Geometry check sheet. Reference: the model listing, model coordinates, mm. Face numbers are marked on the shaded views. Round coordinates to 2 decimals unless told otherwise and drop trailing zeros. Loops run counter-clockwise (first coordinate to the right, second up) from the corner with the lowest first, then second, coordinate; pieces in that order, holes last.
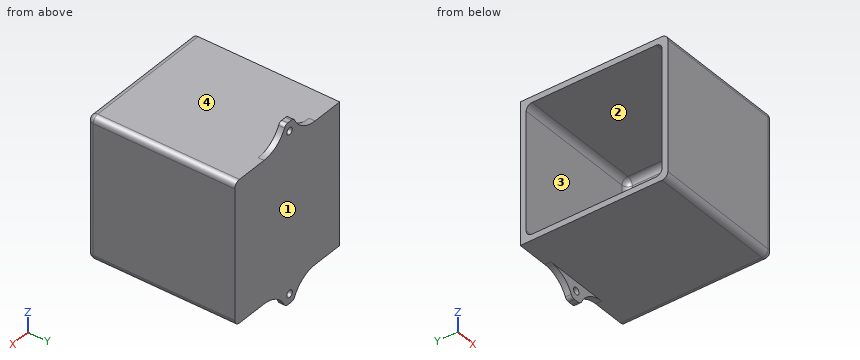
```python
from build123d import *

# Parameters (mm, degrees)
SKETCH1_W           = 60
SKETCH1_H           = 60
BOSS_EXTRUDE1_DEPTH = 60
SHELL1_T            = -2.5
SKETCH5_R           = 1.5
BOSS_EXTRUDE3_DEPTH = 2.5
SKETCH6_W           = 60
SKETCH6_H           = 60
BOSS_EXTRUDE4_DEPTH = 2.5
SKETCH7_W           = 60
SKETCH7_H           = 62.5
CUT_EXTRUDE1_DEPTH  = 2.5
FILLET4_R           = 2.5
FILLET5_R           = 12.5
FILLET6_R           = 2.5


with BuildPart() as part:
    # Sketch1 → Boss-Extrude1 (new body)
    with BuildSketch(Plane(origin=(0, 0, 0), x_dir=(1, 0, 0), z_dir=(0, 1, 0))):
        with Locations((30, 30)):
            Rectangle(SKETCH1_W, SKETCH1_H)
    extrude(amount=BOSS_EXTRUDE1_DEPTH)

    # Shell1
    shell1_openings = [part.faces().sort_by_distance(p)[0] for p in [
        (30, 0, -30),
    ]]
    offset(amount=SHELL1_T, openings=shell1_openings, kind=Kind.INTERSECTION)

    # Sketch5 → Boss-Extrude3 (add)
    # profile 1 of 2: a face of its own
    with BuildSketch(Plane(origin=(0, 60, 0), x_dir=(1, 0, 0), z_dir=(0, 1, 0))):
        with BuildLine():
            Line((27, 60), (27, 66))
            ThreePointArc((27, 66), (27.585786438, 67.414213562), (29, 68))
            Line((29, 68), (31, 68))
            ThreePointArc((31, 68), (32.414213562, 67.414213562), (33, 66))
            Line((33, 66), (33, 60))
            Line((33, 60), (27, 60))
        make_face()
        with Locations(Location((30, 64, 0), (0, 0, 270))):
            Circle(SKETCH5_R, mode=Mode.SUBTRACT)
    # profile 2 of 2: a face of its own
    with BuildSketch(Plane(origin=(0, 60, 0), x_dir=(1, 0, 0), z_dir=(0, 1, 0))):
        with BuildLine():
            Line((33, 0), (27, 0))
            Line((27, 0), (27, -6))
            ThreePointArc((27, -6), (27.585786438, -7.414213562), (29, -8))
            Line((29, -8), (31, -8))
            ThreePointArc((31, -8), (32.414213562, -7.414213562), (33, -6))
            Line((33, -6), (33, 0))
        make_face()
        with Locations(Location((30, -4, 0), (0, 0, 90))):
            Circle(SKETCH5_R, mode=Mode.SUBTRACT)
    extrude(amount=-BOSS_EXTRUDE3_DEPTH)

    # Sketch6 → Boss-Extrude4 (add)
    with BuildSketch(Plane.XZ):
        with Locations((30, -30)):
            Rectangle(SKETCH6_W, SKETCH6_H)
    extrude(amount=BOSS_EXTRUDE4_DEPTH)

    # Sketch7 → Cut-Extrude1 (cut)
    with BuildSketch(Plane.ZY):
        with Locations((-30, 28.75)):
            Rectangle(SKETCH7_W, SKETCH7_H)
    extrude(amount=-CUT_EXTRUDE1_DEPTH, mode=Mode.SUBTRACT)

    # Fillet4
    fillet4_edges = [part.edges().sort_by_distance(p)[0] for p in [
        (31.25, -2.5, 0),
        (60, -2.5, -30),
        (31.25, -2.5, -60),
        (60, 28.75, -60),
        (60, 28.75, 0),
    ]]
    fillet(fillet4_edges, radius=FILLET4_R)

    # Fillet5
    # the kernel refuses this fillet: 12.5 mm, written as the material it adds along each edge
    with BuildSketch(Plane(origin=(27, 60, 0), x_dir=(-1, 0, 0), z_dir=(0, -1, 0)), Plane(origin=(33, 60, -60), x_dir=(1, 0, 0), z_dir=(0, -1, 0))) as fillet5_piece_1:
        with BuildLine():
            CenterArc((10.961481397, -12.5), FILLET5_R, 90, 63.366881251)
            Line((-0.212209463, -6.896551724), (-1.329578548, -6.336206897))
            ThreePointArc((-1.329578548, -6.336206897), (-1.25, -6), (-1.25, 0))
            Line((-1.25, 0), (0, 1.25))
            Line((0, 1.25), (10.961481397, 1.25))
            Line((10.961481397, 1.25), (10.961481397, 0))
        make_face()
    extrude(amount=2.5)
    with BuildSketch(Plane(origin=(33, 60, 0), x_dir=(1, 0, 0), z_dir=(0, -1, 0)), Plane(origin=(27, 60, -60), x_dir=(-1, 0, 0), z_dir=(0, -1, 0))) as fillet5_piece_2:
        with BuildLine():
            CenterArc((10.961481397, 12.5), FILLET5_R, 206.633118749, 63.366881251)
            Line((-0.212209463, 6.896551724), (-1.329578548, 6.336206897))
            ThreePointArc((-1.329578548, 6.336206897), (-1.25, 6), (-1.25, 0))
            Line((-1.25, 0), (0, -1.25))
            Line((0, -1.25), (10.961481397, -1.25))
            Line((10.961481397, -1.25), (10.961481397, 0))
        make_face()
    extrude(amount=2.5)

    # Fillet6
    fillet6_edges = [part.edges().sort_by_distance(p)[0] for p in [
        (30, 0, -2.5),
        (57.5, 0, -30),
        (57.5, 28.75, -2.5),
        (30, 0, -57.5),
        (57.5, 28.75, -57.5),
        (30, 57.5, -2.5),
        (57.5, 57.5, -30),
        (30, 57.5, -57.5),
    ]]
    fillet(fillet6_edges, radius=FILLET6_R)


solid = part.part
```
1) Scan lines: line 1 along Y through (x, z) = (26, -21.5); line 2 along Z through (x, y) = (21, 5.5); line 3 along X through (y, z) = (3, -12). Record each from-to range of solid material in increasing order.
Report:
line 1: y = -2.5 to 0, 57.5 to 60
line 2: z = -60 to -57.5, -2.5 to 0
line 3: x = 57.5 to 60
2) Mould release check, pull along Z, two halves, no side actions. Record for the marked faces 1, 2, 3 and 4: +Z half, -Z half, draft (parallel to the pull), parting line (faces both ways), or undercut.
Report:
face 1: draft
face 2: undercut
face 3: undercut
face 4: +Z half
3) Sectioned sample at C-C, the plane x = 49. Record the cut outline in (y, z).
Report:
outline: (-2.5, -57.5) arc R2.5 ccw to (0, -60) - (60, -60) - (60, 0) - (0, 0) arc R2.5 ccw to (-2.5, -2.5) - close; hole (0, -55) arc R2.5 ccw to (2.5, -57.5) - (55, -57.5) arc R2.5 ccw to (57.5, -55) - (57.5, -5) arc R2.5 ccw to (55, -2.5) - (2.5, -2.5) arc R2.5 ccw to (0, -5) - close
4) Gauge pin test, flat ends, axial feed: pin 1 (5 mm diameter, centred on x = 30, z = 4, fed in from -Y); pin 2 (16.5 mm diameter, centred on x = 32.5, y = 37, fed in from +Z); pin 3 (25 mm diameter, centred on y = 40, z = -26, fed in from -X); pin 4 (1.8 mm diameter, centred on x = 30, z = -64, fed in from -Y). Record the tip position at first contact, or that the pin passes through.
Report:
pin 1: stops at y = 57.5
pin 2: stops at z = 0
pin 3: stops at x = 57.5
pin 4: passes through
5) Sectioned sample at D-D, the plane z = -32. Record the cut outline in (x, y).
Report:
outline: (2.5, -2.5) - (57.5, -2.5) arc R2.5 ccw to (60, 0) - (60, 60) - (2.5, 60) - (2.5, 57.5) - (55, 57.5) arc R2.5 cw to (57.5, 55) - (57.5, 2.5) arc R2.5 cw to (55, 0) - (2.5, 0) - close
6) Sectioned sample at B-B, the plane y = 43.5. Record the cut outline in (x, z).
Report:
outline: (2.5, -60) - (57.5, -60) arc R2.5 ccw to (60, -57.5) - (60, -2.5) arc R2.5 ccw to (57.5, 0) - (2.5, 0) - (2.5, -2.5) - (55, -2.5) arc R2.5 cw to (57.5, -5) - (57.5, -55) arc R2.5 cw to (55, -57.5) - (2.5, -57.5) - close
7) Sectioned sample at A-A, the plane x = 30. Record the cut outline in (y, z), then the cut area to 3 significant figures.
Report:
outline: (-2.5, -57.5) arc R2.5 ccw to (0, -60) - (57.5, -60) - (57.5, -62.5) - (60, -62.5) - (60, 2.5) - (57.5, 2.5) - (57.5, 0) - (0, 0) arc R2.5 ccw to (-2.5, -2.5) - close; (57.5, -68) - (60, -68) - (60, -65.5) - (57.5, -65.5) - close; (57.5, 5.5) - (60, 5.5) - (60, 8) - (57.5, 8) - close; hole (0, -55) arc R2.5 ccw to (2.5, -57.5) - (55, -57.5) arc R2.5 ccw to (57.5, -55) - (57.5, -5) arc R2.5 ccw to (55, -2.5) - (2.5, -2.5) arc R2.5 ccw to (0, -5) - close
area: 615 mm2
